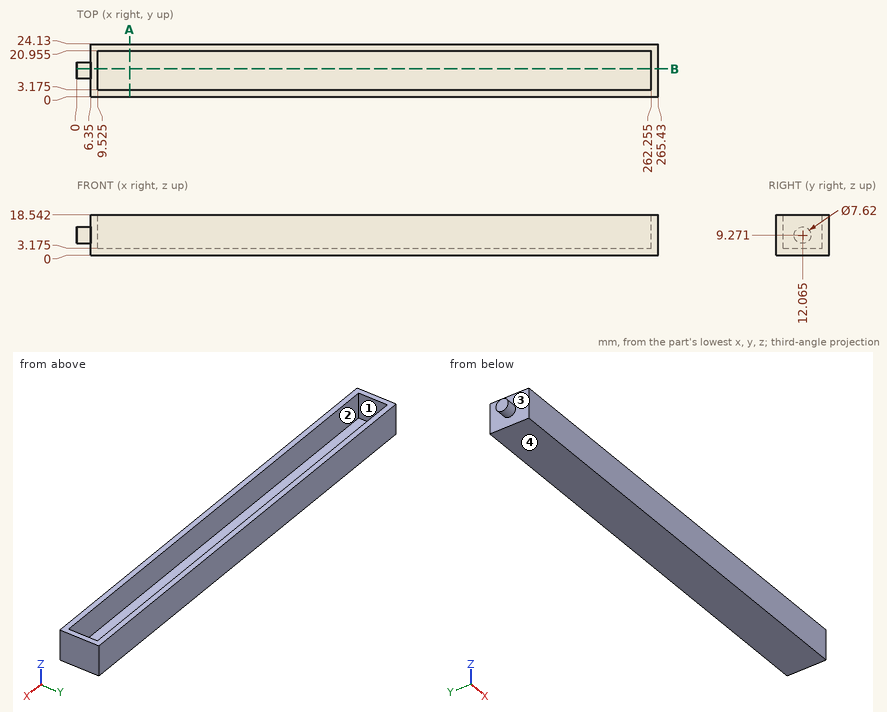
Print and shaded views of the part. All mm, measured from the part's lowest x, y and z. Round coordinates to 2 decimals unless told otherwise and drop trailing zeros. Write each loop counter-clockwise with the first axis right and the second up, starting at its lowest first coordinate (ties: lowest second). Pieces come first, ordered by that corner, then holes.
(1) Slice it at B-B, the plane y = 12.75. Write the cut outline in (x, z) (3 decimals), and give its area (3 significant figures).
(2) Probe line 1 along X through (y, z) = (5.5, 9.5) (3 decimals); line 2 along X through (y, z) = (9, 10) (3 decimals); line 3 along Y through (x, z) = (86, 17) (3 decimals). List the from-to ranges inside material, lowest first.
(3) Mould opens along X. For the marked faces 1, 2, 3 and 4 say: pulls with the +X half, pulls with the -X half, needs draft (parallel to the pull), parting line crosses it, or undercut.
(4) Slice it at A-A, the plane x = 24. Write the cut outline in (y, z) (3 decimals).
(5) Drop flat-ended pins along their axis: P1, Ø2, axis at x = 68.5, y = 9.5, coming from the +Z side (3 decimals); P2, Ø1.5, axis at y = 13.5, z = 2.5, coming from the -X side. Give the stop position or say it passes through.
From the geometry:
1. outline: (0, 5.523) - (6.35, 5.523) - (6.35, 0) - (265.43, 0) - (265.43, 18.542) - (262.255, 18.542) - (262.255, 3.175) - (9.525, 3.175) - (9.525, 18.542) - (6.35, 18.542) - (6.35, 13.019) - (0, 13.019) - close
1. area: 968 mm2
2. line 1: x = 6.35 to 9.525, 262.255 to 265.43
2. line 2: x = 0 to 9.525, 262.255 to 265.43
2. line 3: y = 0 to 3.175, 20.955 to 24.13
3. face 1: undercut
3. face 2: undercut
3. face 3: pulls with the -X half
3. face 4: needs draft
4. outline: (0, 0) - (24.13, 0) - (24.13, 18.542) - (20.955, 18.542) - (20.955, 3.175) - (3.175, 3.175) - (3.175, 18.542) - (0, 18.542) - close
5. P1: stops at z = 3.175
5. P2: stops at x = 6.35
